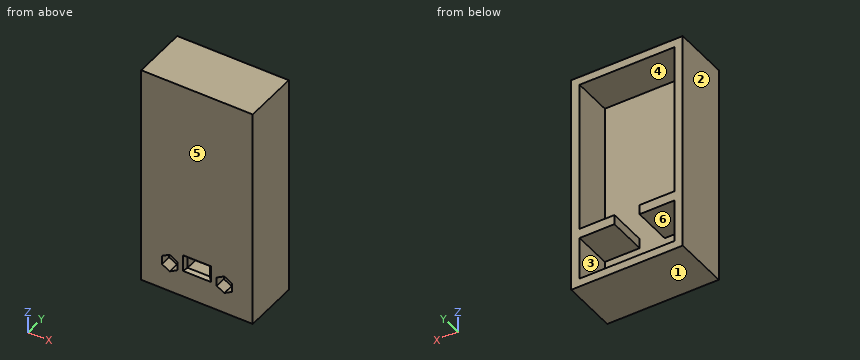
from build123d import *

# Parameters (mm, degrees)
SKETCH1_W                = 40
SKETCH1_H                = 80
SKETCH1_R                = 1.5
SKETCH1_W_2              = 8
SKETCH1_H_2              = 4
INITIAL_EXTRUDE_DEPTH    = 20
MAIN_START               = 6
MAIN_CAVITY_DEPTH        = 43.989794856
SKETCH1_4_R              = 1.5
NUT_CAPTURE_BOTTOM_DEPTH = 4
SENSOR_HOLE_CHAMFER_SIZE = 1
SKETCH3_W                = 16
SKETCH3_H                = 3
GPIO_CUTOUT_SENSOR_DEPTH = 3


with BuildPart() as part:
    # Sketch1 → Initial Extrude (new body)
    with BuildSketch(Plane(origin=(0, 0, 0), x_dir=(1, 0, 0), z_dir=(0, 1, 0))):
        Rectangle(SKETCH1_W, SKETCH1_H)
        with Locations(Location((-9.800487558, 29.300592934, 0), (0, 0, 270))):
            Circle(SKETCH1_R, mode=Mode.SUBTRACT)
        with Locations(Location((9.800487558, 29.300592934, 0), (0, 0, 270))):
            Circle(SKETCH1_R, mode=Mode.SUBTRACT)
        with Locations((0, 27.300592934)):
            Rectangle(SKETCH1_W_2, SKETCH1_H_2, mode=Mode.SUBTRACT)
    extrude(amount=INITIAL_EXTRUDE_DEPTH)

    # Sketch1_3 → Main Cavity (cut, through all)
    with BuildSketch(Plane(origin=(0, 0, 0), x_dir=(1, 0, 0), z_dir=(0, 1, 0)).offset(MAIN_START)):
        Polygon((17, -37), (-17, -37), (-17, 18), (-4.5, 18), (-4.5, 21.5), (-17, 21.5), (-17, 37), (17, 37), (17, 21.5), (4.5, 21.5), (4.5, 18), (17, 18), align=None)
    extrude(amount=MAIN_CAVITY_DEPTH, mode=Mode.SUBTRACT)

    # Sketch1_4 → Nut Capture Bottom (cut)
    # profile 1 of 2: a face of its own
    with BuildSketch(Plane(origin=(0, 0, 0), x_dir=(1, 0, 0), z_dir=(0, 1, 0))):
        Polygon((12.550487558, 27.712879693), (12.550487558, 30.888306174), (9.800487558, 32.476019414), (7.050487558, 30.888306174), (7.050487558, 27.712879693), (9.800487558, 26.125166453), align=None)
        with Locations(Location((9.800487558, 29.300592934, 0), (0, 0, 270))):
            Circle(SKETCH1_4_R, mode=Mode.SUBTRACT)
    # profile 2 of 2: a face of its own
    with BuildSketch(Plane(origin=(0, 0, 0), x_dir=(1, 0, 0), z_dir=(0, 1, 0))):
        Polygon((-7.050487558, 27.712879693), (-7.050487558, 30.888306174), (-9.800487558, 32.476019414), (-12.550487558, 30.888306174), (-12.550487558, 27.712879693), (-9.800487558, 26.125166453), align=None)
        with Locations(Location((-9.800487558, 29.300592934, 0), (0, 0, 270))):
            Circle(SKETCH1_4_R, mode=Mode.SUBTRACT)
    extrude(amount=NUT_CAPTURE_BOTTOM_DEPTH, mode=Mode.SUBTRACT)

    # Sensor Hole Chamfer
    sensor_hole_chamfer_edges = [part.edges().sort_by_distance(p)[0] for p in [
        (0, 0, -29.300592934),
        (-4, 0, -27.300592934),
        (0, 0, -25.300592934),
        (4, 0, -27.300592934),
    ]]
    chamfer(sensor_hole_chamfer_edges, length=SENSOR_HOLE_CHAMFER_SIZE)

    # Sketch3 → GPIO Cutout Sensor (cut)
    with BuildSketch(Plane(origin=(0, 6, 0), x_dir=(1, 0, 0), z_dir=(0, 1, 0))):
        with Locations((0, 33.5)):
            Rectangle(SKETCH3_W, SKETCH3_H)
    extrude(amount=-GPIO_CUTOUT_SENSOR_DEPTH, mode=Mode.SUBTRACT)


solid = part.part
Can you work these out from the model? Positions are in its coordinate system, mm. Face numbers are marked on the shaded views. A direction names the side the tool comes from. Round coordinates to 2 decimals unless told otherwise and drop trailing zeros. Order: outer loops, then holes, each group sorted by start corner. A loop starts at its lowest first (then second) coordinate and runs counter-clockwise, first axis right, second up. Notation, with made-up numbers: M -19.5,47.25 L -2.5,47.25 A27 cw -2.5,67.25 Z; hole C -17,38.25 d6. An arc over 180 degrees is marked long. Use a Markdown table: item, result.
1) Imagine slicing it at C-C (y = 2.25). List the corners of the cut face in (x, z) for me.
Geometry says:
| item | result |
|---|---|
| outline | M -20,-40 L 20,-40 L 20,40 L -20,40 Z; hole M -12.55,-30.89 L -9.8,-32.48 L -7.05,-30.89 L -7.05,-27.71 L -9.8,-26.13 L -12.55,-27.71 Z; hole M -4,-29.3 L 4,-29.3 L 4,-25.3 L -4,-25.3 Z; hole M 7.05,-30.89 L 9.8,-32.48 L 12.55,-30.89 L 12.55,-27.71 L 9.8,-26.13 L 7.05,-27.71 Z |
2) If we mould it in two halves opening along X, with no side actions, what happens to the marked faces 1, 2, 3 and 4? For each: +X half, -X half, draft (parallel to the pull), parting line (faces both ways), or undercut.
Geometry says:
| item | result |
|---|---|
| face 1 | draft |
| face 2 | -X half |
| face 3 | undercut |
| face 4 | undercut |
3) I'm going to push flat-ended pins straight in: P1, Ø4, axis at x = -9.8, z = -29.3, coming from the -Y side; P2, Ø2.5, axis at x = 2, z = -34, coming from the +Y side; P3, Ø6, axis at x = 10.5, z = -30.5, coming from the -Y side. Where does each tip first touch, or does it pass through?
Geometry says:
| item | result |
|---|---|
| P1 | stops at y = 4 |
| P2 | stops at y = 6 |
| P3 | stops at y = 0 |
4) If I drill on line 1 along Z through (x, y) = (5, 15); line 2 along Z through (x, y) = (-3.5, 17.5); line 3 along X through (y, z) = (11.25, 3), over which ranges is the centre line in solid material (lowest first)?
Geometry says:
| item | result |
|---|---|
| line 1 | z = -40 to -37, -21.5 to -18, 37 to 40 |
| line 2 | z = -40 to -37, 37 to 40 |
| line 3 | x = -20 to -17, 17 to 20 |
5) Imagine slicing it at D-D (z = 19). List the corners of the cut face in (x, y) for me, then the cut area to 3 significant figures.
Geometry says:
| item | result |
|---|---|
| outline | M -20,0 L 20,0 L 20,20 L 17,20 L 17,6 L -17,6 L -17,20 L -20,20 Z |
| area | 324 mm² |
6) Imagine slicing it at A-A (x = -1). List the corners of the cut face in (y, z) for me, then the cut area to 3 significant figures.
Geometry says:
| item | result |
|---|---|
| outline | M 0,-40 L 20,-40 L 20,-37 L 6,-37 L 6,-35 L 3,-35 L 3,-32 L 6,-32 L 6,-29.3 L 1,-29.3 L 0,-30.3 Z; M 0,-24.3 L 1,-25.3 L 6,-25.3 L 6,37 L 20,37 L 20,40 L 0,40 Z |
| area | 530 mm² |
7) On a 3-axis mill with a long thin cutter (end or side, diameter ignored), from which of +Z, -Z, +X, -X, +Y, -Y can I reach the whole of each face in a straight line? I mean the marked faces 5 and 6. Say none if no direction works.
Geometry says:
| item | result |
|---|---|
| face 5 | +Z, -Z, +X, -X, -Y |
| face 6 | +Y |
8) Imagine slicing it at B-B (y = 14.75). List the corners of the cut face in (x, z) for me.
Geometry says:
| item | result |
|---|---|
| outline | M -20,-40 L 20,-40 L 20,40 L -20,40 Z; hole M -17,-37 L 17,-37 L 17,-21.5 L 4.5,-21.5 L 4.5,-18 L 17,-18 L 17,37 L -17,37 L -17,-18 L -4.5,-18 L -4.5,-21.5 L -17,-21.5 Z |
